Geometry: final body of the model. Coordinates: model frame, mm. Face numbers are marked on the shaded views. A direction names the side the tool comes from. Coordinates: 2 decimals unless noted, no trailing zeros. Order: outer loops, then holes, each group sorted by start corner. A loop starts at its lowest first (then second) coordinate and runs counter-clockwise, first axis right, second up. Notation, with made-up numbers: M 78,74 L 87,74 A25 cw 87,90 Z; hole C 81.25,-4 d3. An arc over 180 degrees is marked long. Write item = value, one per line.
from build123d import *

# Parameters (mm, degrees)
SKETCH_R              = 25
PAD_DEPTH             = 12.5
SKETCH001_W           = 6.2
SKETCH001_H           = 6.2
PAD001_DEPTH          = 23
CHAMFER_ANGLE         = 70
CHAMFER_SIZE          = 1.2
POCKET_DEPTH          = 171.715492
POLARPATTERN_COUNT    = 8
CHAMFER001_SIZE       = 0.8
SKETCH004_R           = 5.5
POCKET001_DEPTH       = 165.840033
POLARPATTERN001_COUNT = 5


with BuildPart() as part:
    # Sketch → Pad (new body)
    with BuildSketch(Plane.XY):
        Circle(SKETCH_R)
    extrude(amount=PAD_DEPTH)

    # Sketch001 → Pad001 (join)
    with BuildSketch(Plane.XY):
        Rectangle(SKETCH001_W, SKETCH001_H)
    extrude(amount=PAD001_DEPTH)

    # Chamfer
    chamfer_edges = [part.edges().sort_by_distance(p)[0] for p in [
        (0, -3.1, 12.5),
        (3.1, 0, 12.5),
        (0, 3.1, 12.5),
        (-3.1, 0, 12.5),
    ]]
    chamfer_side = part.faces().sort_by_distance((-24.292893, 0, 12.5))[0]
    chamfer(chamfer_edges, length=CHAMFER_SIZE, angle=CHAMFER_ANGLE, reference=chamfer_side)

    # Sketch002 → Pocket (cut, through all)
    with BuildSketch(Plane.XY):
        with BuildLine():
            ThreePointArc((-15, 37), (0, 22), (15, 37))
            Line((-15, 37), (15, 37))
        make_face()
    pocket = extrude(amount=POCKET_DEPTH, mode=Mode.SUBTRACT)

    # PolarPattern: Pocket ×8 about axis
    polarpattern_axis = Axis((0, 0, 0), (0, 0, 1))
    for i in range(1, POLARPATTERN_COUNT):
        add(pocket.rotate(polarpattern_axis, i * 360 / POLARPATTERN_COUNT), mode=Mode.SUBTRACT)

    # Sketch003 → Groove (revolve, cut)
    with BuildSketch(Plane.XZ):
        Polygon((7.66865, 25.207804), (7.66865, 13.637294), (28.54884, 7.5), (28.54884, 25.207804), align=None)
    revolve(axis=Axis((0, 0, 0), (0, 0, 1)), mode=Mode.SUBTRACT)

    # Chamfer001
    chamfer001_edges = [part.edges().sort_by_distance(p)[0] for p in [
        (0, 3.1, 23),
        (3.1, 0, 23),
        (0, -3.1, 23),
        (-3.1, 0, 23),
    ]]
    chamfer(chamfer001_edges, length=CHAMFER001_SIZE)

    # Sketch004 → Pocket001 (cut, through all)
    with BuildSketch(Plane.XY):
        with Locations((0, 14)):
            Circle(SKETCH004_R)
    pocket001 = extrude(amount=POCKET001_DEPTH, mode=Mode.SUBTRACT)

    # PolarPattern001: Pocket001 ×5 about axis
    polarpattern001_axis = Axis((0, 0, 0), (0, 0, 1))
    for i in range(1, POLARPATTERN001_COUNT):
        add(pocket001.rotate(polarpattern001_axis, i * 360 / POLARPATTERN001_COUNT), mode=Mode.SUBTRACT)


solid = part.part
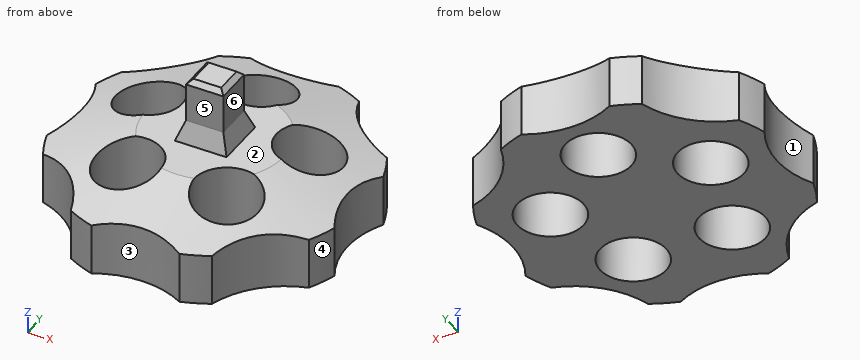
1) Section A-A, the plane x = 0. Return loops of the section in (y, z), and give its area (3 significant figures).
Numbers:
outline = M -22,0 L 8.5,0 L 8.5,12.5 L 4.3,12.5 L 3.1,15.8 L 3.1,22.2 L 2.3,23 L -2.3,23 L -3.1,22.2 L -3.1,15.8 L -4.3,12.5 L -11.54,12.5 L -22,9.42 Z; M 19.5,0 L 22,0 L 22,9.42 L 19.5,10.16 Z
area = 458 mm²
2) Set-up query: the marked faces 4, 5 and 6. Return all of +Z, -Z, +X, -X, +Y, -Y with unobstructed straight access to the full face (end or side cutting, diameter ignored); none if empty.
Numbers:
face_4 = +Z, -Z, +X, -Y
face_5 = +Z, +X, -X, -Y
face_6 = +Z, +X, +Y, -Y
3) Section B-B, the plane y = 0. Return loops of the section in (x, z).
Numbers:
outline = M -22,0 L -16.71,0 L -16.71,10.98 L -22,9.42 Z; M -9.92,0 L 9.92,0 L 9.92,12.5 L 4.3,12.5 L 3.1,15.8 L 3.1,22.2 L 2.3,23 L -2.3,23 L -3.1,22.2 L -3.1,15.8 L -4.3,12.5 L -9.92,12.5 Z; M 16.71,0 L 22,0 L 22,9.42 L 16.71,10.98 Z
4) Line query: L1, parallel to Y at x = 0, z = 6.5; L2, parallel to X at y = -14, z = 2; L3, parallel to X at y = 5.5, z = 3.75. Output: solid intervals per line, ascending.
Numbers:
L1 = -22 to 8.5, 19.5 to 22
L2 = -17.38 to -13.04, -3.42 to 3.42, 13.04 to 17.38
L3 = -23.04 to -18.69, -7.94 to 7.94, 18.69 to 23.04
5) Mould query, pull axis Y, two halves, no side actions, for the marked faces 1, 2 and 3. Classes: pulls with the +Y half, pulls with the -Y half, needs draft (parallel to the pull), parting line crosses it, or undercut.
Numbers:
face_1 = undercut
face_2 = needs draft
face_3 = pulls with the -Y half
6) Pin query (flat end, axial travel): pin 1 (3 mm diameter, centred on x = 0, z = 18.5, fed in from +Y); pin 2 (7 mm diameter, centred on y = -1.5, z = 19.5, fed in from +X); pin 3 (5 mm diameter, centred on x = -11.5, y = 2.5, fed in from +Z); pin 4 (17.5 mm diameter, centred on x = -13.31, y = 4.33, fed in from -Z). Return the tip coordinate at first contact, or that it passes through.
Numbers:
pin_1 = 3.1
pin_2 = 3.1
pin_3 = through
pin_4 = 0
7) Section C-C, the plane z = 17.75. Return loops of the section in (x, y), and give its area (3 significant figures).
Numbers:
outline = M -3.1,-3.1 L 3.1,-3.1 L 3.1,3.1 L -3.1,3.1 Z
area = 38.4 mm²
8) Section D-D, the plane y = -9.5. Give the number of separate pieces and of enclosed holes in the cut face, and give its area (3 significant figures).
Numbers:
separate_pieces = 3
enclosed_holes = 0
area = 267 mm²
